Can you work these out from the model? Positions are in its coordinate system, mm. A direction names the side the tool comes from. Give positions to 0.01 mm unless a question says otherwise; leave off trailing zeros. Write each loop counter-clockwise with the first axis right and the second up, starting at its lowest first coordinate (ties: lowest second). Pieces come first, ordered by that corner, then holes.
from build123d import *

# Parameters (mm, degrees)
F0_R     = 245
F1_DEPTH = 880
F2_R     = 10
F3_T     = -7.62


with BuildPart() as f1:
    # F0 (on Top) → F1 (new body)
    with BuildSketch(Plane.XY):
        Circle(F0_R)
    extrude(amount=-F1_DEPTH)

    # F2
    f2_edges = [f1.edges().sort_by_distance(p)[0] for p in [
        (-245, 0, -880),
    ]]
    fillet(f2_edges, radius=F2_R)

    # F3
    f3_openings = [f1.faces().sort_by_distance(p)[0] for p in [
        (0, 0, 0),
    ]]
    offset(amount=F3_T, openings=f3_openings)


solid = f1.part
(1) Will these pins go through, and if not, where does the flat tip stop? P1, Ø1.5, axis at y = 8, z = -129.5, coming from the +X side; P2, Ø10, axis at x = 13.5, y = -143.5, coming from the +Z side; P3, Ø1, axis at x = 26, z = -342, coming from the -Y side.
Returned:
P1: stops at x = 244.89
P2: stops at z = -872.38
P3: stops at y = -243.67
(2) If I drill on L1, parallel to X at y = 1, z = -714; L2, parallel to Y at x = 4, z = -833.5, over which ranges is the centre line in solid material (lowest first)?
Returned:
L1: x = -245 to -237.38, 237.38 to 245
L2: y = -244.97 to -237.35, 237.35 to 244.97
(3) Imagine slicing it at A-A, the plane y = 0. Write out the boundary of the cut face in (x, z), plus the area to 3 significant figures.
Returned:
outline: (-245, -870) arc R10 ccw to (-235, -880) - (235, -880) arc R10 ccw to (245, -870) - (245, 0) - (237.38, 0) - (237.38, -870) arc R2.38 cw to (235, -872.38) - (-235, -872.38) arc R2.38 cw to (-237.38, -870) - (-237.38, 0) - (-245, 0) - close
area: 17,000 mm2
(4) For faces 4 (the face through (-3, 3, -872.38)), 5 (the face through (-128, 201, 0)), which set-ups out of +Z, -Z, +X, -X, +Y, -Y let a thin tool reach every point of the face, with its end or its side?
Returned:
face 4: +Z
face 5: +Z, +X, -X, +Y, -Y
(5) Imagine slicing it at B-B, the plane z = -314.5. Write out the boundary of the cut face in (x, y), plus the area to 3 significant figures.
Returned:
outline: circle Ø490 at (0, 0); hole circle Ø474.76 at (0, 0)
area: 11,500 mm2
(6) If we mould it in two halves opening along X, with no side actions, what happens to faces 1 (the face through (-3, 3, -880)), 2 (the face through (-53.111, -239.174, -428.91)), 3 (the face through (-188.38, -144.44, -428.91))? For each: +X half, -X half, draft (parallel to the pull), parting line (faces both ways), or undercut.
Returned:
face 1: draft
face 2: parting line
face 3: undercut
